Work out the finished part from the listing and answer in its coordinate system (mm). Coordinates: 2 decimals unless noted, no trailing zeros. Order: outer loops, then holes, each group sorted by start corner. A loop starts at its lowest first (then second) coordinate and runs counter-clockwise, first axis right, second up. Notation, with made-up numbers: (-4, 12.5) -> (2, 12.5) arc R24 ccw to (2, 27.5) -> close; hole circle Ø10 at (-29.5, 32.25). An arc over 180 degrees is marked (long way). Write item = value, one per line. Start each with the question number.
Q1. The part is cut by section D-D, the plane x = 7.25. Determine the outline of the cut face in (y, z), plus the area to 3 significant figures.
Q2. Straight lines are drawn through the part: L1, parallel to X at y = 6.5, z = 0; L2, parallel to Y at x = 8, z = -4; L3, parallel to X at y = -1, z = -2.25. For each, find the intervals that lie inside material, in ascending order. Write a range as from..to.
Q3. Flat-ended cylindrical pins translate along their axes: pin 1 (6 mm diameter, centred on x = 5.5, y = 1.5, fed in from +Z); pin 2 (6 mm diameter, centred on y = 10, z = 4, fed in from -X). Find the tip coordinate at first contact, or state that the pin passes through.
Q4. The part is cut by section A-A, the plane x = 0. Determine the outline of the cut face in (y, z).
Q5. For a pull along Y with two mould halves and no side action, classify faces 1 (the flat face through (-2, -2, 2)), 2 (the cylindrical face through (-2.44, 4.9, -0.54)), 3 (the flat face through (-2, 12, 2)), 4 (the cylindrical face through (-7.81, 4.93, -1.73)) as +Y half, -Y half, draft (parallel to the pull), parting line (faces both ways), or undercut.
Q6. The part is cut by section B-B, the plane z = 0. Determine the outline of the cut face in (x, y), plus the area to 3 significant figures.
Q7. The part is cut by section C-C, the plane z = 6.5. Determine the outline of the cut face in (x, y).
```python
from build123d import *

# Parameters (mm, degrees)
SKETCH_1_R      = 8
SKETCH_1_R_2    = 2.5
EXTRUDE_1_DEPTH = 10
EXTRUDE_START   = -2
SKETCH_1_3_R    = 9
SKETCH_1_3_R_2  = 8
SKETCH_1_3_R_3  = 2.5
EXTRUDE_2_DEPTH = 2
EXTRUDE_START_2 = 10
SKETCH_1_4_R    = 9
SKETCH_1_4_R_2  = 8
SKETCH_1_4_R_3  = 2.5
EXTRUDE_3_DEPTH = 2


with BuildPart() as part:
    # 草图1 → 凸台-拉伸1 (new body)
    with BuildSketch(Plane(origin=(0, 0, 0), x_dir=(1, 0, 0), z_dir=(0, 1, 0))):
        with Locations(Location((0, 0, 0), (0, 0, 270))):
            Circle(SKETCH_1_R)
        with Locations(Location((0, 0, 0), (0, 0, 270))):
            Circle(SKETCH_1_R_2, mode=Mode.SUBTRACT)
    extrude(amount=EXTRUDE_1_DEPTH)

    # 草图1<3> → 凸台-拉伸2 (add)
    # profile 1 of 2: a face of its own
    with BuildSketch(Plane(origin=(0, 0, 0), x_dir=(1, 0, 0), z_dir=(0, 1, 0)).offset(EXTRUDE_START)):
        with Locations(Location((0, 0, 0), (0, 0, 270))):
            Circle(SKETCH_1_3_R)
        with Locations(Location((0, 0, 0), (0, 0, 270))):
            Circle(SKETCH_1_3_R_2, mode=Mode.SUBTRACT)
    # profile 2 of 2: a face of its own
    with BuildSketch(Plane(origin=(0, 0, 0), x_dir=(1, 0, 0), z_dir=(0, 1, 0)).offset(EXTRUDE_START)):
        with Locations(Location((0, 0, 0), (0, 0, 270))):
            Circle(SKETCH_1_3_R_2)
        with Locations(Location((0, 0, 0), (0, 0, 270))):
            Circle(SKETCH_1_3_R_3, mode=Mode.SUBTRACT)
    extrude(amount=EXTRUDE_2_DEPTH)

    # 草图1<4> → 凸台-拉伸3 (add)
    # profile 1 of 2: a face of its own
    with BuildSketch(Plane(origin=(0, 0, 0), x_dir=(1, 0, 0), z_dir=(0, 1, 0)).offset(EXTRUDE_START_2)):
        with Locations(Location((0, 0, 0), (0, 0, 270))):
            Circle(SKETCH_1_4_R)
        with Locations(Location((0, 0, 0), (0, 0, 270))):
            Circle(SKETCH_1_4_R_2, mode=Mode.SUBTRACT)
    # profile 2 of 2: a face of its own
    with BuildSketch(Plane(origin=(0, 0, 0), x_dir=(1, 0, 0), z_dir=(0, 1, 0)).offset(EXTRUDE_START_2)):
        with Locations(Location((0, 0, 0), (0, 0, 270))):
            Circle(SKETCH_1_4_R_2)
        with Locations(Location((0, 0, 0), (0, 0, 270))):
            Circle(SKETCH_1_4_R_3, mode=Mode.SUBTRACT)
    extrude(amount=EXTRUDE_3_DEPTH)


solid = part.part
```
Model answer:
q1.outline = (-2, -5.33) -> (0, -5.33) -> (0, -3.38) -> (10, -3.38) -> (10, -5.33) -> (12, -5.33) -> (12, 5.33) -> (10, 5.33) -> (10, 3.38) -> (0, 3.38) -> (0, 5.33) -> (-2, 5.33) -> close
q1.area = 110 mm2
q2.L1 = -8..-2.5, 2.5..8
q2.L2 = -2..0, 10..12
q2.L3 = -8.71..-1.09, 1.09..8.71
q3.pin_1 = 8.52
q3.pin_2 = -8.94
q4.outline = (-2, -9) -> (0, -9) -> (0, -8) -> (10, -8) -> (10, -9) -> (12, -9) -> (12, -2.5) -> (-2, -2.5) -> close; (-2, 2.5) -> (12, 2.5) -> (12, 9) -> (10, 9) -> (10, 8) -> (0, 8) -> (0, 9) -> (-2, 9) -> close
q5.face_1 = -Y half
q5.face_2 = draft
q5.face_3 = +Y half
q5.face_4 = undercut
q6.outline = (-9, -2) -> (-2.5, -2) -> (-2.5, 12) -> (-9, 12) -> (-9, 10) -> (-8, 10) -> (-8, 0) -> (-9, 0) -> close; (2.5, -2) -> (9, -2) -> (9, 0) -> (8, 0) -> (8, 10) -> (9, 10) -> (9, 12) -> (2.5, 12) -> close
q6.area = 162 mm2
q7.outline = (-6.22, -2) -> (6.22, -2) -> (6.22, 0) -> (4.66, 0) -> (4.66, 10) -> (6.22, 10) -> (6.22, 12) -> (-6.22, 12) -> (-6.22, 10) -> (-4.66, 10) -> (-4.66, 0) -> (-6.22, 0) -> close
